Source: CAD feature listing. Evaluate the final solid. Frame: model axes, mm. Face numbers are marked on the shaded views. A direction names the side the tool comes from. Give positions to 0.01 mm unless a question says otherwise; leave off trailing zeros. Order: outer loops, then holes, each group sorted by start corner. A loop starts at its lowest first (then second) coordinate and runs counter-clockwise, first axis right, second up.
from build123d import *

# Parameters (mm, degrees)
BOSS_EXTRUDE1_DEPTH      = 60
BOSS_EXTRUDE1_DEPTH_BACK = 60
SKETCH2_R                = 1.5
CUT_EXTRUDE1_DEPTH       = 5


with BuildPart() as part:
    # Sketch1 → Boss-Extrude1 (new body, two sides)
    with BuildSketch(Plane.XY) as boss_extrude1_sk:
        Polygon((-34.15, 4), (-34.15, 65.3), (34.15, 65.3), (34.15, 4), (49.15, 4), (49.15, 0), (34.15, 0), (30.15, 0), (30.15, 60.3), (-30.15, 60.3), (-30.15, 0), (-34.15, 0), (-49.15, 0), (-49.15, 4), align=None)
    extrude(amount=BOSS_EXTRUDE1_DEPTH)
    extrude(boss_extrude1_sk.sketch, amount=-BOSS_EXTRUDE1_DEPTH_BACK)

    # Sketch2 → Cut-Extrude1 (cut, through all)
    with BuildSketch(Plane(origin=(0, 4, 0), x_dir=(1, 0, 0), z_dir=(0, 1, 0))):
        with Locations((41.946567631, -31.148436051)):
            Circle(SKETCH2_R)
        with Locations((41.946567631, 8.851563949)):
            Circle(SKETCH2_R)
        with Locations((41.946567631, 48.851563949)):
            Circle(SKETCH2_R)
    cut_extrude1 = extrude(amount=-CUT_EXTRUDE1_DEPTH, mode=Mode.SUBTRACT)

    # Mirror1: Cut-Extrude1 across plane
    add(cut_extrude1.mirror(Plane(origin=(0, 0, 0), x_dir=(0, 0, 1), z_dir=(1, 0, 0))), mode=Mode.SUBTRACT)


solid = part.part
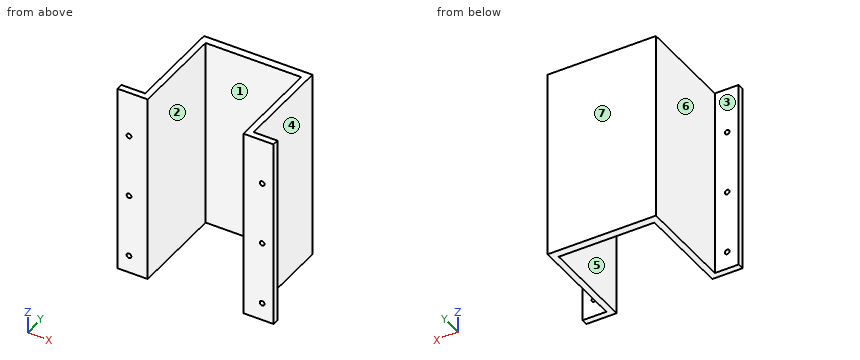
1) Reachability of the marked faces 5, 6 and 7 from +Z, -Z, +X, -X, +Y, -Y: full face, straight path, thin tool, end or side. Return the list, or none.
Checks:
face 5: +Z, -Z, -Y
face 6: +Z, -Z, -X, +Y
face 7: +Z, -Z, +X, -X, +Y
2) Ray query, L1, parallel to X at y = 23.5, z = 13; L2, parallel to Y at x = -42, z = -22.5; L3, parallel to Y at x = -7, z = 0.5. Return the intervals inside material, ascending.
Checks:
L1: x = -34.15 to -30.15, 30.15 to 34.15
L2: y = 0 to 4
L3: y = 60.3 to 65.3
3) Section query B-B on z = 49. Output: boundary loops of the cut face in (x, y).
Checks:
outline: (-49.15, 0) - (-30.15, 0) - (-30.15, 60.3) - (30.15, 60.3) - (30.15, 0) - (49.15, 0) - (49.15, 4) - (34.15, 4) - (34.15, 65.3) - (-34.15, 65.3) - (-34.15, 4) - (-49.15, 4) - close
4) Section query D-D on x = -17. Output: boundary loops of the cut face in (y, z).
Checks:
outline: (60.3, -60) - (65.3, -60) - (65.3, 60) - (60.3, 60) - close
5) Section query C-C on x = 36. Output: boundary loops of the cut face in (y, z), and give its area (3 significant figures).
Checks:
outline: (0, -60) - (4, -60) - (4, 60) - (0, 60) - close
area: 480 mm2
6) Pull-direction query (X, two-part tool) for the marked faces 1, 2, 3 and 4; classes: +X half, -X half, draft (parallel to the pull), parting line (faces both ways), or undercut.
Checks:
face 1: undercut
face 2: undercut
face 3: draft
face 4: +X half
7) First-contact query: pin 1 Ø10 at (y, z) = (33, -1) entering from +X; pin 2 Ø5 at (x, z) = (-41.95, -8.85) entering from -Y; pin 3 Ø2 at (x, z) = (-37.5, 22) entering from +Y. Flat tips, straight axial feed; report the tip coordinate or a pass-through.
Checks:
pin 1: stops at x = 34.15
pin 2: stops at y = 0
pin 3: stops at y = 4
8) Section query A-A on y = 40. Output: boundary loops of the cut face in (x, z), and give its area (3 significant figures).
Checks:
outline: (-34.15, -60) - (-30.15, -60) - (-30.15, 60) - (-34.15, 60) - close; (30.15, -60) - (34.15, -60) - (34.15, 60) - (30.15, 60) - close
area: 960 mm2
